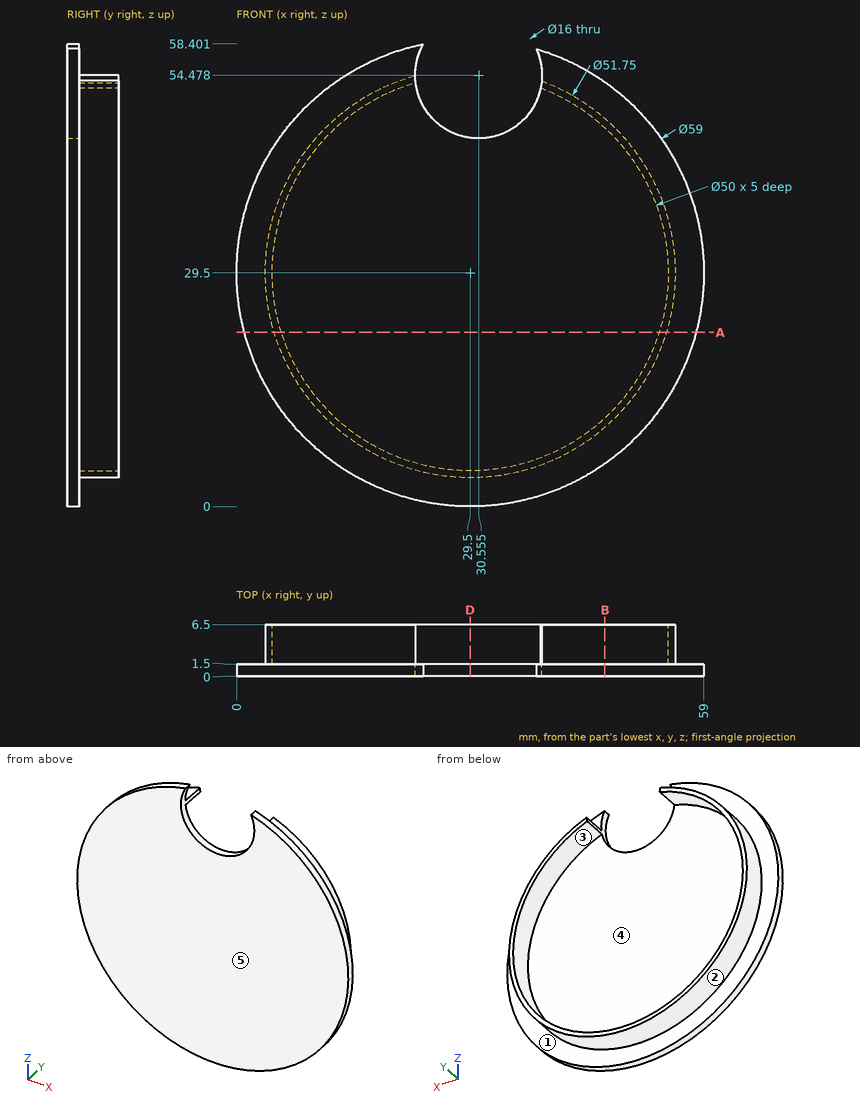
Input: dimensioned drawing with shaded views. Units: mm. Origin: part minimum x, y, z. A direction names the side the tool comes from. Coordinates: 2 decimals unless noted, no trailing zeros. Order: outer loops, then holes, each group sorted by start corner. A loop starts at its lowest first (then second) coordinate and runs counter-clockwise, first axis right, second up. Notation, with made-up numbers: (-34, 42) - (20, 42) arc R15 ccw to (20, 53) - close; hole circle Ø1 at (-15.5, 45.25). An arc over 180 degrees is marked (long way). Put each result on its own line as item: value.
1. Cut plane B-B on x = 46.5. Return the cut outline in (y, z).
Report:
outline: (0, 5.39) - (1.5, 5.39) - (1.5, 9.99) - (6.5, 9.99) - (6.5, 11.17) - (1.5, 11.17) - (1.5, 47.83) - (6.5, 47.83) - (6.5, 49.01) - (1.5, 49.01) - (1.5, 53.61) - (0, 53.61) - close
2. Cut plane D-D on x = 29.5. Return the cut outline in (y, z) (1 decimal).
Report:
outline: (0, 0) - (1.5, 0) - (1.5, 3.6) - (6.5, 3.6) - (6.5, 4.5) - (1.5, 4.5) - (1.5, 46.5) - (0, 46.5) - close
3. Draft query along X for the marked faces 1, 2 and 3. Return one class per face: pulls with the +X half, pulls with the -X half, needs draft (parallel to the pull), parting line crosses it, or undercut.
Report:
face 1: needs draft
face 2: parting line crosses it
face 3: undercut
4. Cut plane A-A on z = 22. Return the cut outline in (x, y) (1 decimal).
Report:
outline: (1, 0) - (58, 0) - (58, 1.5) - (54.3, 1.5) - (54.3, 6.5) - (53.3, 6.5) - (53.3, 1.5) - (5.7, 1.5) - (5.7, 6.5) - (4.7, 6.5) - (4.7, 1.5) - (1, 1.5) - close
5. Contact query for flat-ended pins moving along their axis: pin 1 Ø1.5 at (x, y) = (25.5, 4.5) entering from +Z (1 decimal); pin 2 Ø1.5 at (x, z) = (12, 26.5) entering from +Y; pin 3 Ø1.5 at (x, y) = (16.5, 2.5) entering from +Z. Output: stop coordinate, or through.
Report:
pin 1: stops at z = 5
pin 2: stops at y = 1.5
pin 3: stops at z = 52.29
6. Line query: line 1 along X through (y, z) = (5.05, 29.5) (1 decimal); line 2 along Z through (x, y) = (29.5, 3) (1 decimal); line 3 along Y through (x, z) = (37.5, 30.5). Output: solid intervals per line, ascending.
Report:
line 1: x = 3.6 to 4.5, 54.5 to 55.4
line 2: z = 3.6 to 4.5
line 3: y = 0 to 1.5
7. Reachability of the marked faces 4 and 5 from +Z, -Z, +X, -X, +Y, -Y: full face, straight path, thin tool, end or side. Return the list, or none.
Report:
face 4: +Y
face 5: +Z, -Z, +X, -X, -Y
